Autodesk Inventor part; units mm, degrees
ref_plane "YZ Plane" through (0, 0, 0) normal (1, 0, 0) x (0, 1, 0)
ref_plane "XZ Plane" through (0, 0, 0) normal (0, 1, 0) x (-1, 0, 0)
ref_plane "XY Plane" through (0, 0, 0) normal (0, 0, 1) x (1, 0, 0)
sketch "Sketch1" plane through (0, 0, 0) normal (0, 1, 0) x (-1, 0, 0)
  line L0 (0, 0) -> (609.6, 0)
  line L1 (609.6, 0) -> (609.6, -304.8)
  line L2 (609.6, -304.8) -> (0, -304.8)
  line L3 (0, -304.8) -> (0, 0)
  dimension "d0" = 304.8
  dimension "d1" = 609.6
extrude "Extrusion1" add sketch "Sketch1" along normal blind 3.175
sketch "Sketch2" plane through (0, 3.175, 0) normal (0, 1, 0) x (1, 0, 0)
  line L0 (-609.6, 0) -> (0, 0)
  line L1 (0, 0) -> (0, 304.8)
  line L2 (-609.6, 0) -> (0, 0)
  line L3 (0, 0) -> (0, 304.8)
  line L4 (0, 304.8) -> (-609.6, 304.8)
  line L5 (-609.6, 304.8) -> (-609.6, 0)
  line L6 (-606.425, 3.175) -> (-3.175, 3.175)
  line L7 (-3.175, 3.175) -> (-3.175, 301.625)
  line L8 (-3.175, 301.625) -> (-606.425, 301.625)
  line L9 (-606.425, 301.625) -> (-606.425, 3.175)
  dimension "d4" = 3.175
  dimension "d5" = 3.175
  dimension "d6" = 3.175
  dimension "d7" = 3.175
extrude "Extrusion2" add sketch "Sketch2" along normal blind 301.625
sketch "Sketch5" plane through (0, 0, 0) normal (1, 0, 0) x (0, 0, -1)
  circle A0 centre (152.4, 38.1) radius 12.7
  line L0 (304.8, 0) -> (0, 0)
  line L1 (304.8, 0) -> (304.8, 304.8)
  dimension "d18" = 25.4
  dimension "d19" = 38.1
  dimension "d20" = 152.4
extrude "Extrusion5" cut sketch "Sketch5" against normal blind 25.4
properties part number "Burner"
Work out the finished part from the listing and answer in its coordinate system (mm). A direction names the side the tool comes from. Give positions to 0.01 mm unless a question says otherwise; leave off trailing zeros. Write each loop counter-clockwise with the first axis right and the second up, starting at its lowest first coordinate (ties: lowest second). Pieces come first, ordered by that corner, then holes. Notation, with made-up numbers: (-22, 14) - (-6, 14) arc R23 ccw to (-6, 43) - close; hole circle Ø4 at (71.25, 45). An arc over 180 degrees is marked (long way). Use one line per item in the form item = value.
1. A cutting plane is placed at C-C (x = -251.5). Write down the section's boundary in (y, z) (3 decimals), and give its area (3 significant figures).
Filled in:
outline = (0, -304.8) - (304.8, -304.8) - (304.8, -301.625) - (3.175, -301.625) - (3.175, -3.175) - (304.8, -3.175) - (304.8, 0) - (0, 0) - close
area = 2,880 mm^2
2. For faces 1 (the face through (-309, 152, -3.175)), 2 (the face through (0, 150, -155)), determine the directions among +Z, -Z, +X, -X, +Y, -Y from which every point of the face is accessible in a straight line to the end or side of a thin tool.
Filled in:
face_1 = +Y
face_2 = +Z, -Z, +X, +Y, -Y
3. A cutting plane is placed at B-B (y = 202.5). Write down the section's boundary in (x, z) (3 decimals).
Filled in:
outline = (-609.6, -304.8) - (0, -304.8) - (0, 0) - (-609.6, 0) - close; hole (-606.425, -301.625) - (-3.175, -301.625) - (-3.175, -3.175) - (-606.425, -3.175) - close
4. Consider L1, parallel to X at y = 36, z = -202 (3 decimals); L2, parallel to Z at x = -215, y = 100 (3 decimals); L3, parallel to Y at x = -1.7, z = -152.4. Determine where each line is inside the solid, lowest interval first.
Filled in:
L1 = -609.6 to -606.425, -3.175 to 0
L2 = -304.8 to -301.625, -3.175 to 0
L3 = 0 to 25.4, 50.8 to 304.8
5. This flat-tipped pin is pushed along its axis until it touches: pin 1 Ø1.5 at (x, z) = (-404, -161.5) entering from +Y (3 decimals). Where does it stop, or does it pass through?
Filled in:
pin_1 = 3.175
6. A cutting plane is placed at D-D (y = 38.1). Write down the section's boundary in (x, z) (3 decimals).
Filled in:
outline = (-609.6, -304.8) - (0, -304.8) - (0, -165.1) - (-3.175, -165.1) - (-3.175, -301.625) - (-606.425, -301.625) - (-606.425, -3.175) - (-3.175, -3.175) - (-3.175, -139.7) - (0, -139.7) - (0, 0) - (-609.6, 0) - close
7. A cutting plane is placed at A-A (z = -152.4). Write down the section's boundary in (x, y) (3 decimals), and give its area (3 significant figures).
Filled in:
outline = (-609.6, 0) - (0, 0) - (0, 25.4) - (-3.175, 25.4) - (-3.175, 3.175) - (-606.425, 3.175) - (-606.425, 304.8) - (-609.6, 304.8) - close; (-3.175, 50.8) - (0, 50.8) - (0, 304.8) - (-3.175, 304.8) - close
area = 3,770 mm^2
8. Determine the mould class of faces 3 (the face through (-301, 0, -150)), 4 (the face through (-1.565, 46.683, -143.04)), 5 (the face through (-609.6, 150, -150)), 6 (the face through (-301, 3.175, -150)) for opening direction Y: released by +Y, released by -Y, zero draft, split by the parting line, or undercut.
Filled in:
face_3 = released by -Y
face_4 = undercut
face_5 = zero draft
face_6 = released by +Y
